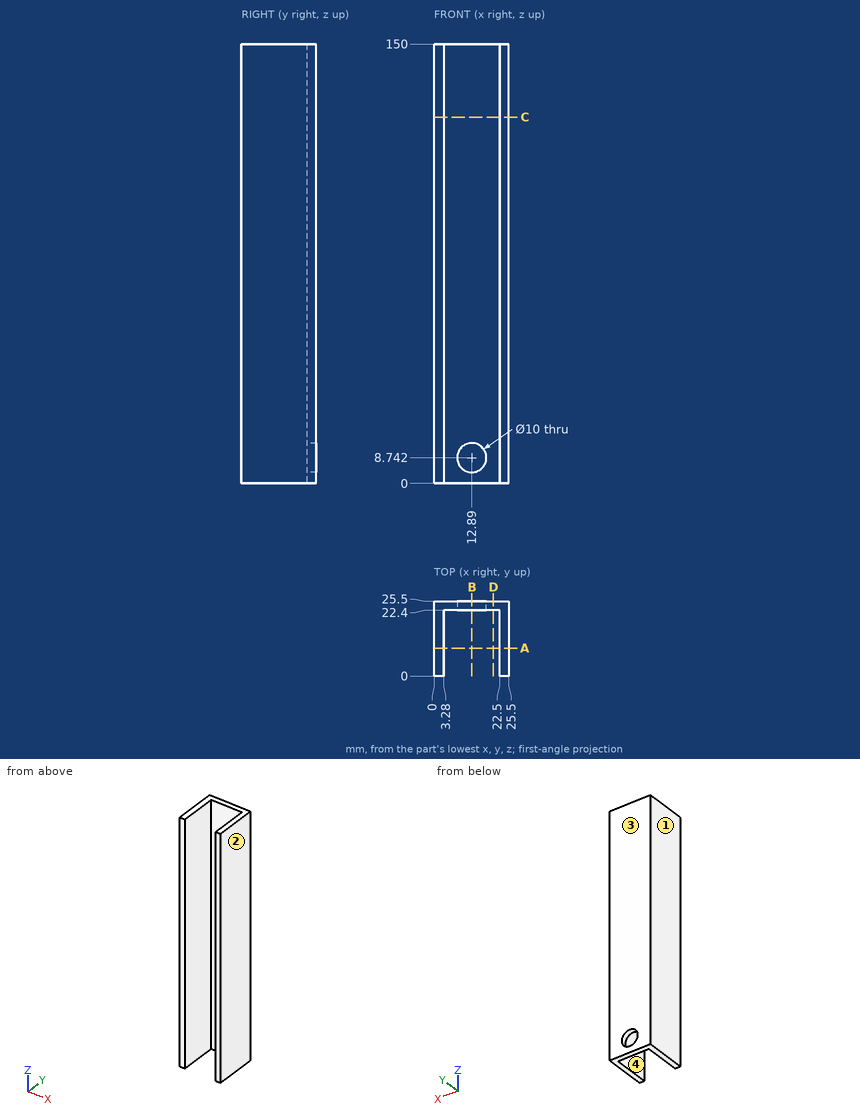
The drawing under review shows one solid part. Ordinate dimensions are in mm from its lowest x, y, z. Round coordinates to 2 decimals unless told otherwise and drop trailing zeros. Write each loop counter-clockwise with the first axis right and the second up, starting at its lowest first coordinate (ties: lowest second). Pieces come first, ordered by that corner, then holes.
(1) We need section C-C on z = 125. Give the boundary of the cut face in (x, y), and give its area (3 significant figures).
(2) Insertion check: pin 1 (9.5 mm diameter, centred on x = 9.5, z = 45, fed in from -Y); pin 2 (1.5 mm diameter, centred on y = 5, z = 80, fed in from -X); pin 3 (6 mm diameter, centred on x = 8, y = 14.5, fed in from -Z). Each pin has a flat end and moves straight along its axis. Give the tip position at first contact, or say it passes through.
(3) We need section D-D on x = 20.25. Give the boundary of the cut face in (y, z).
(4) Mouldability with a two-part tool opening along X and no side actions: class the marked faces 1, 2, 3 and 4 as +X half, -X half, draft (parallel to the pull), parting line (faces both ways), or undercut.
(5) Wall thickness on L1, parallel to X at y = 14, z = 142; L2, parallel to Z at x = 12.89, y = 24.75; L3, parallel to Y at x = 17, z = 106: over which ranges is each line inside the solid? List them lowest first.
(6) We need section A-A on y = 9.5. Give the boundary of the cut face in (x, z), and give its area (3 significant figures).
(7) We need section B-B on x = 12.89. Give the boundary of the cut face in (y, z).
Findings below:
1. outline: (0, 0) - (3.28, 0) - (3.28, 22.4) - (22.5, 22.4) - (22.5, 0) - (25.5, 0) - (25.5, 25.5) - (0, 25.5) - close
1. area: 220 mm2
2. pin 1: stops at y = 22.4
2. pin 2: stops at x = 0
2. pin 3: passes through
3. outline: (22.4, 0) - (25.5, 0) - (25.5, 150) - (22.4, 150) - close
4. face 1: -X half
4. face 2: +X half
4. face 3: draft
4. face 4: undercut
5. L1: x = 0 to 3.28, 22.5 to 25.5
5. L2: z = 0 to 3.74, 13.74 to 150
5. L3: y = 22.4 to 25.5
6. outline: (0, 0) - (3.28, 0) - (3.28, 150) - (0, 150) - close; (22.5, 0) - (25.5, 0) - (25.5, 150) - (22.5, 150) - close
6. area: 942 mm2
7. outline: (22.4, 0) - (25.5, 0) - (25.5, 3.74) - (22.4, 3.74) - close; (22.4, 13.74) - (25.5, 13.74) - (25.5, 150) - (22.4, 150) - close
